from build123d import *

# Parameters (mm, degrees)
F0_R     = 1.651
F1_DEPTH = 2


# Not quite as in the source:
# - ends of sketch curves that miss each other by under 0.0002 mm in the source are joined


with BuildPart() as f1:
    # F0 (on Front) → F1 (new body)
    with BuildSketch(Plane.XZ):
        with BuildLine():
            Line((7.937499, 23.216594), (7.937501, 39.751))
            ThreePointArc((7.937501, 39.751), (3.975101, 43.7134), (0.012701, 39.751))
            Line((0.012701, 39.751), (0.0127, 28.556342))
            ThreePointArc((0.0127, 28.556342), (-0.524833277, 25.999444372), (-2.046427009, 23.8754340098))
            ThreePointArc((-2.046427009, 23.8754340098), (-5.7457403837, 19.2987254647), (-7.9375015933, 13.8372821405))
            Line((-7.9375015933, 13.8372821405), (-2.222499, -37.1094))
            Line((-2.222499, -37.1094), (0.574712, -41.785211))
            ThreePointArc((0.574712, -41.785211), (6.0796125104, -43.1083226832), (7.2879037085, -37.5770851913))
            Line((7.2879037085, -37.5770851913), (4.000105, -32.566839))
            ThreePointArc((4.000105, -32.566839), (3.2819142622, -31.0818977846), (2.97042001, -29.4620769994))
            Line((2.97042001, -29.4620769994), (0.692124, 8.634151))
            ThreePointArc((0.692124, 8.634151), (1.7368417824, 13.9147568002), (5.2269018653, 18.0130141926))
            ThreePointArc((5.2269018653, 18.0130141926), (7.2192261395, 20.2829710591), (7.937499, 23.216594))
        make_face()
        with Locations((3.975094, -39.751)):
            Circle(F0_R, mode=Mode.SUBTRACT)
        with Locations((3.975101, 39.751)):
            Circle(F0_R, mode=Mode.SUBTRACT)
    extrude(amount=F1_DEPTH)


solid = f1.part
Verification items for the finished model (mm, model axes). A direction names the side the tool comes from. Round coordinates to 2 decimals unless told otherwise and drop trailing zeros. Loops run counter-clockwise (first coordinate to the right, second up) from the corner with the lowest first, then second, coordinate; pieces in that order, holes last. Notation, with made-up numbers: M 67.25,46 L 72.25,46 A16 ccw 72.25,60 Z; hole C 67.5,21 d8. An arc over 180 degrees is marked long. Write each question's results on one line, items separated by ' | '.
1) Scan lines: L1, parallel to Z at x = 4.5, y = -1; L2, parallel to Z at x = 6.75, y = -0.1; L3, parallel to X at y = -0.4, z = 31.5. Record each from-to range of solid material in increasing order. Write a range as from..to.
Checks:
L1: z = -43.68..-41.32, -38.19..-33.33, 17.46..38.19, 41.32..43.68 | L2: z = -42.58..-36.76, 19.52..42.58 | L3: x = 0.01..7.94
2) Section check C-C on z = -0.5. Record the boundary of the cut face in (x, y).
Checks:
outline: M -6.33,-2 L 1.24,-2 L 1.24,0 L -6.33,0 Z
3) Gauge pin test, flat end, axial feed: P1, Ø2, axis at x = 4, z = 15.5, coming from the +Y side. Record the tip position at first contact, or that the pin passes through.
Checks:
P1: passes through
4) Section check A-A on y = -1.55. Record the boundary of the cut face in (x, z).
Checks:
outline: M -7.94,13.84 L -2.22,-37.11 L 0.57,-41.79 A3.96 ccw long 7.29,-37.58 L 4,-32.57 A6.35 cw 2.97,-29.46 L 0.69,8.63 A10.67 cw 5.23,18.01 A6.35 ccw 7.94,23.22 L 7.94,39.75 A3.96 ccw 0.01,39.75 L 0.01,28.56 A6.35 cw -2.05,23.88 A19.81 ccw Z; hole C 3.98,-39.75 d3.3; hole C 3.98,39.75 d3.3
5) Section check B-B on x = -6. Record the boundary of the cut face in (y, z), then the cut area to 3 significant figures.
Checks:
outline: M -2,-3.43 L 0,-3.43 L 0,18.85 L -2,18.85 Z | area: 44.6 mm2
6) Access from +Z, -Z, +X, -X, +Y, -Y to the whole of each face (thin tool, end or side, straight path). Record for faces 1 (the flat face through (0, -2, 1)), 2 (the flat face through (5.67, -0.99, -35.11)), 3 (the flat face through (0.013, -1, 34)).
Checks:
face 1: +Z, -Z, +X, -X, -Y | face 2: +X, +Y, -Y | face 3: +Z, -X, +Y, -Y
7) Mould release check, pull along Z, two halves, no side actions. Record for faces 4 (the flat face through (0, 0, 1)), 5 (the flat face through (1.847, -0.986, -10.681)), 6 (the flat face through (-5.12, -0.99, -11.28)): released by +Z, released by -Z, zero draft, split by the parting line, or undercut.
Checks:
face 4: zero draft | face 5: undercut | face 6: released by -Z
